```python
from build123d import *

# Parameters (mm, degrees)
SKETCH_2_W               = 1.6
SKETCH_2_H               = 1
CUT_EXTRUDE_1_DEPTH      = 4
CUT_EXTRUDE_1_DEPTH_BACK = 4
CHAMFER_1_SIZE           = 0.6


with BuildPart() as part:
    # Эскиз1 → Повернуть1 (revolve)
    with BuildSketch(Plane(origin=(0, 0, 0), x_dir=(1, 0, 0), z_dir=(0, 1, 0))):
        Polygon((0, 0), (-3, 0), (-3, 14.700961894), (-0.75, 16), (0, 16), align=None)
    revolve(axis=Axis((0, 0, -16), (0, 0, 1)))

    # Эскиз2 → Вырез-Вытянуть1 (cut, two sides)
    with BuildSketch(Plane(origin=(0, 0, 0), x_dir=(0, 0, -1), z_dir=(1, 0, 0))) as cut_extrude_1_sk:
        with Locations((0.8, 0)):
            Rectangle(SKETCH_2_W, SKETCH_2_H)
    extrude(amount=CUT_EXTRUDE_1_DEPTH, mode=Mode.SUBTRACT)
    extrude(cut_extrude_1_sk.sketch, amount=-CUT_EXTRUDE_1_DEPTH_BACK, mode=Mode.SUBTRACT)

    # Фаска1
    chamfer_1_edges = [part.edges().sort_by_distance(p)[0] for p in [
        (0, 3, 0),
        (0, -3, 0),
    ]]
    chamfer(chamfer_1_edges, length=CHAMFER_1_SIZE)


solid = part.part
```
Read the model definition and answer for the solid it produces. Units are mm, in the model's axes. A direction names the side the tool comes from. Coordinates: 2 decimals unless noted, no trailing zeros. Order: outer loops, then holes, each group sorted by start corner. A loop starts at its lowest first (then second) coordinate and runs counter-clockwise, first axis right, second up. Notation, with made-up numbers: (-33.75, -29) - (17.25, -29) arc R28 cw to (17.25, 7) - close; hole circle Ø4 at (7.5, -24). An arc over 180 degrees is marked (long way). Answer as a JSON object with one key per item and string values. Group by question number.
Item 1: Section C-C (z = -4) is taken. Give the vertices of the cut face in (x, y), plus the area to 3 significant figures.
Item 2: The mould has two halves that part along Y. Classify faces 1 (the face through (-0.1, -2.6, -0.2)), 2 (the face through (0, -0.5, -1)), 3 (the face through (0, 0, -16)): +Y half, -Y half, draft (parallel to the pull), parting line (faces both ways), or undercut.
Item 3: Section D-D (z = -15) is taken. Give the vertices of the cut face in (x, y), plus the area to 3 significant figures.
Item 4: A tool of negligible diameter and unlimited length cuts with its end or side. For faces 4 (the face through (0, 1, 0)), 5 (the face through (0, 0.5, -1)), from which of +Z, -Z, +X, -X, +Y, -Y can it reach the whole face along a straight path? Write none if from no direction.
Item 5: Consider probe 1 along X at (y, z) = (1.8, -14.5); probe 2 along X at (y, z) = (0.1, -6.5); probe 3 along Y at (x, z) = (0.5, -11). Determine where each line is inside the solid, lowest interval first. Write a range as from..to.
Item 6: Flat-ended cylindrical pins translate along their axes: P1, Ø1, axis at x = -1.5, z = -5, coming from the +Y side; P2, Ø1.5, axis at x = -2, y = 0, coming from the -Z side; P3, Ø2, axis at x = -2, y = 0.5, coming from the +Z side; P4, Ø0.8, axis at x = 1, z = -1, coming from the -Y side. Find the tip coordinate at first contact, or state that the pin passes through.
Item 7: Section A-A (x = 0) is taken. Give the vertices of the cut face in (y, z).
Item 8: Section B-B (y = 0) is taken. Give the vertices of the cut face in (x, z), plus the area to 3 significant figures.
Results are:
{
 "1": {"outline": "circle Ø6 at (0, 0)", "area": "28.3 mm^2"},
 "2": {"face 1": "-Y half", "face 2": "undercut", "face 3": "draft"},
 "3": {"outline": "circle Ø4.96 at (0, 0)", "area": "19.4 mm^2"},
 "4": {"face 4": "+Z, +X, -X, +Y, -Y", "face 5": "+Z, +X, -X"},
 "5": {"probe 1": "x = -2.4..2.4", "probe 2": "x = -3..3", "probe 3": "y = -2.96..2.96"},
 "6": {"P1": "stops at y = 2.83", "P2": "stops at z = -15.71", "P3": "stops at z = 0", "P4": "stops at y = -2.94"},
 "7": {"outline": "(-3, -14.7) - (-0.75, -16) - (0.75, -16) - (3, -14.7) - (3, -0.6) - (2.4, 0) - (0.5, 0) - (0.5, -1.6) - (-0.5, -1.6) - (-0.5, 0) - (-2.4, 0) - (-3, -0.6) - close"},
 "8": {"outline": "(-3, -14.7) - (-0.75, -16) - (0.75, -16) - (3, -14.7) - (3, -1.6) - (-3, -1.6) - close", "area": "83.5 mm^2"}
}
